```python
from build123d import *

# Parameters (mm, degrees)
CROQUIS1_W              = 25.4
CROQUIS1_H              = 31.4
SALIENTE_EXTRUIR1_DEPTH = 2
SALIENTE_EXTRUIR2_START = 1
SALIENTE_EXTRUIR2_DEPTH = 8.4
CROQUIS3_W              = 21.7
CROQUIS3_H              = 29.1
SALIENTE_EXTRUIR3_DEPTH = 19.65
CROQUIS4_W              = 6
CROQUIS4_H              = 0.8
SALIENTE_EXTRUIR4_DEPTH = 9.2
SALIENTE_EXTRUIR5_DEPTH = 11


with BuildPart() as part:
    # Croquis1 → Saliente-Extruir1 (new body)
    with BuildSketch(Plane(origin=(0, 0, 0), x_dir=(1, 0, 0), z_dir=(0, 1, 0))):
        Rectangle(CROQUIS1_W, CROQUIS1_H)
    extrude(amount=SALIENTE_EXTRUIR1_DEPTH)

    # Croquis2 → Saliente-Extruir2 (add)
    with BuildSketch(Plane(origin=(0, 0, 0), x_dir=(0, 0, -1), z_dir=(1, 0, 0)).offset(SALIENTE_EXTRUIR2_START)):
        with BuildLine():
            Line((-11.2, 2), (11.2, 2))
            ThreePointArc((11.2, 2), (2.215809273, 4.278475594), (-5.7, 9.1))
            ThreePointArc((-5.7, 9.1), (-9.165424158, 6.104201813), (-11.2, 2))
        make_face()
    saliente_extruir2 = extrude(amount=SALIENTE_EXTRUIR2_DEPTH)

    # Simetría1: Saliente-Extruir2 across plane
    add(saliente_extruir2.mirror(Plane(origin=(0, 0, 0), x_dir=(0, 0, 1), z_dir=(1, 0, 0))))

    # Croquis3 → Saliente-Extruir3 (add)
    with BuildSketch(Plane.XZ):
        Rectangle(CROQUIS3_W, CROQUIS3_H)
    extrude(amount=SALIENTE_EXTRUIR3_DEPTH)

    # Croquis4 → Saliente-Extruir4 (add)
    with BuildSketch(Plane.XZ.offset(19.65)):
        with Locations((4.75, 10.5)):
            Rectangle(CROQUIS4_W, CROQUIS4_H)
        with Locations((-4.75, 10.5)):
            Rectangle(CROQUIS4_W, CROQUIS4_H)
        with Locations((4.75, 0)):
            Rectangle(CROQUIS4_W, CROQUIS4_H)
        with Locations((4.75, -10.5)):
            Rectangle(CROQUIS4_W, CROQUIS4_H)
        with Locations((-4.75, 0)):
            Rectangle(CROQUIS4_W, CROQUIS4_H)
        with Locations((-4.75, -10.5)):
            Rectangle(CROQUIS4_W, CROQUIS4_H)
    extrude(amount=SALIENTE_EXTRUIR4_DEPTH)

    # Croquis5 → Saliente-Extruir5 (add)
    with BuildSketch(Plane.XZ.offset(19.65)):
        Polygon((0.625, 14.55), (-0.625, 14.55), (-0.625, -4.625), (-10.85, -4.625), (-10.85, -5.875), (-0.625, -5.875), (-0.625, -14.55), (0.625, -14.55), (0.625, -5.875), (10.85, -5.875), (10.85, -4.625), (0.625, -4.625), align=None)
    extrude(amount=SALIENTE_EXTRUIR5_DEPTH)


solid = part.part
```
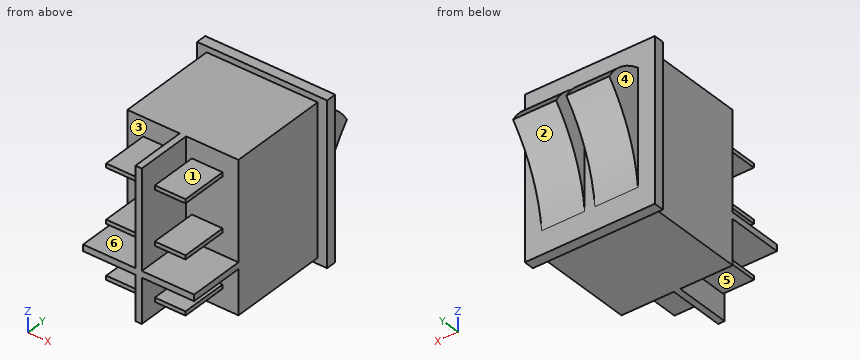
Read the model definition and answer for the solid it produces. Units are mm, in the model's axes. Face numbers are marked on the shaded views. A direction names the side the tool comes from. Give positions to 0.01 mm unless a question says otherwise; leave off trailing zeros. Write each loop counter-clockwise with the first axis right and the second up, starting at its lowest first coordinate (ties: lowest second). Pieces come first, ordered by that corner, then holes. Notation, with made-up numbers: (57, -21) -> (115, -21) arc R27 cw to (115, -4) -> close; hole circle Ø8 at (-10, 13.5). An arc over 180 degrees is marked (long way). Answer as a JSON object with one key per item and string values.
1) Section D-D on y = -8.5 is taken. Write down the section's boundary in (x, z).
Findings below:
{"outline": "(-10.85, -14.55) -> (10.85, -14.55) -> (10.85, 14.55) -> (-10.85, 14.55) -> close"}
2) For a pull along Z with two mould halves and no side action, classify the marked faces 1, 2 and 3 as pulls with the +Z half, pulls with the -Z half, needs draft (parallel to the pull), parting line crosses it, or undercut.
Findings below:
{"face 1": "pulls with the +Z half", "face 2": "pulls with the -Z half", "face 3": "undercut"}
3) Flat-ended cylindrical pins translate along their axes: pin 1 Ø2 at (y, z) = (4, 2) entering from -X; pin 2 Ø12.5 at (x, z) = (-0.5, -5.5) entering from +Y; pin 3 Ø1.8 at (x, y) = (-4.5, -26) entering from -Z. Find the tip coordinate at first contact, or state that the pin passes through.
Findings below:
{"pin 1": "stops at x = -9.4", "pin 2": "stops at y = 5.7", "pin 3": "stops at z = -10.9"}
4) Section C-C on z = -2.5 is taken. Write down the section's boundary in (x, y) (3 decimals), then the cut area to 3 significant figures.
Findings below:
{"outline": "(-12.7, 0) -> (-10.85, 0) -> (-10.85, -19.65) -> (-0.625, -19.65) -> (-0.625, -30.65) -> (0.625, -30.65) -> (0.625, -19.65) -> (10.85, -19.65) -> (10.85, 0) -> (12.7, 0) -> (12.7, 2) -> (9.4, 2) -> (9.4, 4.161) -> (1, 4.161) -> (1, 2) -> (-1, 2) -> (-1, 4.161) -> (-9.4, 4.161) -> (-9.4, 2) -> (-12.7, 2) -> close", "area": "527 mm^2"}
5) A tool of negligible diameter and unlimited length cuts with its end or side. For the marked faces 4, 5 and 6, from which of +Z, -Z, +X, -X, +Y, -Y can it reach the whole face along a straight path? Write none if from no direction.
Findings below:
{"face 4": "+Z, -Z, -X, +Y", "face 5": "-Z, -X, -Y", "face 6": "-X, -Y"}
6) Straight lines are drawn through the part: probe 1 along Z at (x, y) = (7.5, -25.5) (3 decimals); probe 2 along X at (y, z) = (3, -2); probe 3 along Z at (x, y) = (4, -14.5). For each, find the intervals that lie inside material, in ascending order. Write a range as from..to.
Findings below:
{"probe 1": "z = -10.9..-10.1, -5.875..-4.625, -0.4..0.4, 10.1..10.9", "probe 2": "x = -9.4..-1, 1..9.4", "probe 3": "z = -14.55..14.55"}
7) Section B-B on y = -22 is taken. Count the separate pieces of the cut face and the enclosed holes in it, then the cut area to 3 significant figures.
Findings below:
{"separate pieces": "7", "enclosed holes": "0", "area": "90.7 mm^2"}
8) Section A-A on x = -5.5 is taken. Write down the section's boundary in (y, z) (3 decimals), then the cut area to 3 significant figures.
Findings below:
{"outline": "(-30.65, -5.875) -> (-19.65, -5.875) -> (-19.65, -10.1) -> (-28.85, -10.1) -> (-28.85, -10.9) -> (-19.65, -10.9) -> (-19.65, -14.55) -> (0, -14.55) -> (0, -15.7) -> (2, -15.7) -> (2, -11.2) arc R31.144 cw to (9.1, 5.7) arc R11.594 ccw to (2, 11.2) -> (2, 15.7) -> (0, 15.7) -> (0, 14.55) -> (-19.65, 14.55) -> (-19.65, 10.9) -> (-28.85, 10.9) -> (-28.85, 10.1) -> (-19.65, 10.1) -> (-19.65, 0.4) -> (-28.85, 0.4) -> (-28.85, -0.4) -> (-19.65, -0.4) -> (-19.65, -4.625) -> (-30.65, -4.625) -> close", "area": "738 mm^2"}
